Can you work these out from the model? Positions are in its coordinate system, mm. Face numbers are marked on the shaded views. Give positions to 0.01 mm unless a question says otherwise; leave off trailing zeros. Order: outer loops, then holes, each group sorted by start corner. A loop starts at its lowest first (then second) coordinate and runs counter-clockwise, first axis right, second up. Notation, with made-up numbers: M -18.5,17.5 L -7.5,17.5 A32 cw -7.5,43.5 Z; hole C 8,-21 d6. An arc over 180 degrees is marked long. Answer as a JSON object with one key per item and string values.
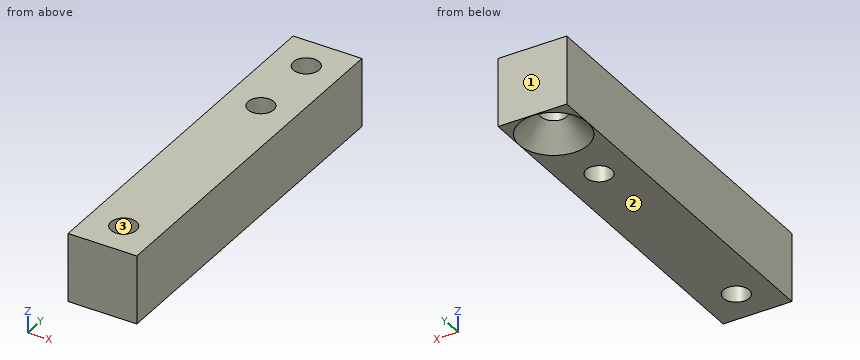
```python
from build123d import *

# Parameters (mm, degrees)
F5_W     = 16
F5_H     = 16
F6_DEPTH = 42.9
F0_R     = 3
F7_DEPTH = 12.5
F2_SIZE  = 4.99999
F3_R     = 3
F4_DEPTH = 16.001


# Not quite as in the source:
# - a fillet or chamfer is up to 0.001 mm smaller than in the source, because OpenCascade refuses the exact size


with BuildPart() as f6:
    # F5 (on Front) → F6 (new body, symmetric)
    with BuildSketch(Plane.XZ):
        Rectangle(F5_W, F5_H)
    extrude(amount=F6_DEPTH, both=True)

    # F0 (on Top) → F7 (cut, symmetric)
    with BuildSketch(Plane.XY):
        with Locations((0, -34.8)):
            Circle(F0_R)
        with Locations((0, 34.8)):
            Circle(F0_R)
    extrude(amount=F7_DEPTH, both=True, mode=Mode.SUBTRACT)

    # F2 (size 5 in the source; OpenCascade refuses exactly that, so slightly less here)
    f2_edges = [f6.edges().sort_by_distance(p)[0] for p in [
        (-3, 34.8, -8),
    ]]
    chamfer(f2_edges, length=F2_SIZE)

    # F3 (on face) → F4 (cut, through all)
    with BuildSketch(Plane.XY.offset(8)):
        with Locations((0, 17.5)):
            Circle(F3_R)
    extrude(amount=-F4_DEPTH, mode=Mode.SUBTRACT)


solid = f6.part
```
1) I want a section at B-B on x = 0. Write out the boundary of the cut face in (y, z), and give its area (3 significant figures).
Results found:
{"outline": "M -42.9,-8 L -37.8,-8 L -37.8,8 L -42.9,8 Z; M -31.8,-8 L 14.5,-8 L 14.5,8 L -31.8,8 Z; M 20.5,-8 L 26.8,-8 L 31.8,-3 L 31.8,8 L 20.5,8 Z; M 37.8,-3 L 42.8,-8 L 42.9,-8 L 42.9,8 L 37.8,8 Z", "area": "1,060 mm²"}
2) I want a section at C-C on z = -4. Write out the boundary of the cut face in (x, y), and give its area (3 significant figures).
Results found:
{"outline": "M -8,-42.9 L 8,-42.9 L 8,42.9 L -8,42.9 Z; hole C 0,34.8 d8; hole C 0,-34.8 d6; hole C 0,17.5 d6", "area": "1,270 mm²"}
3) I need wall thicknesses on L1, parallel to Y at x = 0, z = 3.25; L2, parallel to Y at x = -1.5, z = 5.75; L3, parallel to X at y = -34.8, z = -1.5. Which ranges of each line are inside material? Lowest first, please.
Results found:
{"L1": "y = -42.9 to -37.8, -31.8 to 14.5, 20.5 to 31.8, 37.8 to 42.9", "L2": "y = -42.9 to -37.4, -32.2 to 14.9, 20.1 to 32.2, 37.4 to 42.9", "L3": "x = -8 to -3, 3 to 8"}
4) Thinking about a two-plate mould opening in Y: for the marked faces 1, 2 and 3, which applies, pulls with the +Y half, pulls with the -Y half, needs draft (parallel to the pull), parting line crosses it, or undercut?
Results found:
{"face 1": "pulls with the +Y half", "face 2": "needs draft", "face 3": "undercut"}
5) I'm going to push a flat-ended pin straight in: pin 1 Ø5 at (x, y) = (-2, 30.5) entering from -Z. Where does the tip first touch, or does it pass through?
Results found:
{"pin 1": "stops at z = -7.24"}
6) I want a section at A-A on y = -34.8. Write out the boundary of the cut face in (x, z).
Results found:
{"outline": "M -8,-8 L -3,-8 L -3,8 L -8,8 Z; M 3,-8 L 8,-8 L 8,8 L 3,8 Z"}
